Build history of the part. All positions in model axes, mm. A direction names the side the tool comes from. Round coordinates to 2 decimals unless told otherwise and drop trailing zeros. Write each loop counter-clockwise with the first axis right and the second up, starting at its lowest first coordinate (ties: lowest second). Pieces come first, ordered by that corner, then holes.
1) Which spindle directions (+Z, -Z, +X, -X, +Y, -Y) get a long thin tool onto all of the face, cutting with end or side? Do faces 1 (the flat face through (-6, -2, 29)), 2 (the flat face through (-6, 6, 0)), 3 (the cylindrical face through (8.894, -4.76, 14.703)). Say none if no direction does.
2) Pull direction Y, two halves, no side cores. Call faces 4 (the flat face through (-6, 6, 29)), 5 (the cylindrical face through (-11.106, -4.76, 14.703)), 6 (the cylindrical face through (3.09, 13.91, 14.3)): +Y half, -Y half, draft (parallel to the pull), parting line (faces both ways), or undercut.
3) Saw through at D-D (y = 12.5). Write the cut outline in (x, z), plus the area to 3 significant figures.
4) Flat gauge pins, fed straight in: pin 1 (8 mm diameter, centred on x = 10.5, z = 5.5, fed in from -Y); pin 2 (5 mm diameter, centred on x = 1, y = 11, fed in from -Z); pin 3 (1.5 mm diameter, centred on y = 6.5, z = 9.5, fed in from +X). Where does each tip first touch, or does it go through?
5) Wall check: probe 1 along Y at (x, z) = (0, 10.5); probe 2 along X at (y, z) = (-5, 27); probe 3 along Z at (x, y) = (9, 10.75). Give the ranges that are in metal, low to high.
6) Saw through at B-B (x = -3.5). Write the cut outline in (y, z).
7) Saw through at A-A (y = 0). Write the cut outline in (x, z), plus the area to 4 significant figures.
8) Saw through at C-C (z = 5). Write the cut outline in (x, y), plus the area to 3 significant figures.
from build123d import *

# Parameters (mm, degrees)
SKETCH1_R           = 14.25
SKETCH1_R_2         = 7
BOSS_EXTRUDE1_DEPTH = 29
SKETCH2_R           = 8
SKETCH2_R_2         = 7
BOSS_EXTRUDE2_DEPTH = 1
SKETCH3_R           = 1.5
CUT_EXTRUDE1_DEPTH  = 37.140351409
SKETCH4_R           = 7
SKETCH4_R_2         = 6
BOSS_EXTRUDE3_DEPTH = 29


with BuildPart() as part:
    # Sketch1 → Boss-Extrude1 (new body)
    with BuildSketch(Plane.XY):
        with Locations(Location((0, 0, 0), (0, 0, 180))):
            Circle(SKETCH1_R)
        with Locations(Location((0, 0, 0), (0, 0, 180))):
            Circle(SKETCH1_R_2, mode=Mode.SUBTRACT)
    extrude(amount=BOSS_EXTRUDE1_DEPTH)

    # Sketch2 → Boss-Extrude2 (add)
    with BuildSketch(Plane.XY.offset(29)):
        Circle(SKETCH2_R)
        with Locations(Location((0, 0, 0), (0, 0, 180))):
            Circle(SKETCH2_R_2, mode=Mode.SUBTRACT)
    boss_extrude2 = extrude(amount=BOSS_EXTRUDE2_DEPTH)

    # Mirror1: Boss-Extrude2 across plane
    add(boss_extrude2.mirror(Plane.XY.offset(14.5)))

    # Sketch3 → Cut-Extrude1 (cut, through all)
    with BuildSketch(Plane.XY.offset(29)):
        with Locations((0, 11.547005384)):
            Circle(SKETCH3_R)
        with Locations((10, -5.773502692)):
            Circle(SKETCH3_R)
        with Locations((-10, -5.773502692)):
            Circle(SKETCH3_R)
    extrude(amount=-CUT_EXTRUDE1_DEPTH, mode=Mode.SUBTRACT)

    # Sketch4 → Boss-Extrude3 (add)
    with BuildSketch(Plane.XY.offset(29)):
        with Locations(Location((0, 0, 0), (0, 0, 180))):
            Circle(SKETCH4_R)
        Circle(SKETCH4_R_2, mode=Mode.SUBTRACT)
    extrude(amount=-BOSS_EXTRUDE3_DEPTH)


solid = part.part
Evaluation:
1. face 1: +Z
1. face 2: -Z
1. face 3: +Z, -Z
2. face 4: draft
2. face 5: undercut
2. face 6: parting line
3. outline: (-6.84, 0) - (-1.16, 0) - (-1.16, 29) - (-6.84, 29) - close; (1.16, 0) - (6.84, 0) - (6.84, 29) - (1.16, 29) - close
3. area: 330 mm2
4. pin 1: stops at y = -12.68
4. pin 2: stops at z = 0
4. pin 3: stops at x = 13.04
5. probe 1: y = -14.25 to -6, 6 to 10.05, 13.05 to 14.25
5. probe 2: x = -13.34 to -11.29, -8.71 to -3.32, 3.32 to 8.71, 11.29 to 13.34
5. probe 3: z = 0 to 29
6. outline: (-13.81, 0) - (-7.19, 0) - (-7.19, -1) - (-6.06, -1) - (-6.06, 0) - (-4.87, 0) - (-4.87, 29) - (-6.06, 29) - (-6.06, 30) - (-7.19, 30) - (-7.19, 29) - (-13.81, 29) - close; (4.87, 0) - (6.06, 0) - (6.06, -1) - (7.19, -1) - (7.19, 0) - (13.81, 0) - (13.81, 29) - (7.19, 29) - (7.19, 30) - (6.06, 30) - (6.06, 29) - (4.87, 29) - close
7. outline: (-14.25, 0) - (-8, 0) - (-8, -1) - (-7, -1) - (-7, 0) - (-6, 0) - (-6, 29) - (-7, 29) - (-7, 30) - (-8, 30) - (-8, 29) - (-14.25, 29) - close; (6, 0) - (7, 0) - (7, -1) - (8, -1) - (8, 0) - (14.25, 0) - (14.25, 29) - (8, 29) - (8, 30) - (7, 30) - (7, 29) - (6, 29) - close
7. area: 482.5 mm2
8. outline: circle Ø28.5 at (0, 0); hole circle Ø3 at (-10, -5.77); hole circle Ø12 at (0, 0); hole circle Ø3 at (0, 11.55); hole circle Ø3 at (10, -5.77)
8. area: 504 mm2
